```python
from build123d import *

# Parameters (mm, degrees)
IZIM1_W                     = 30
IZIM1_H                     = 20
Y_KSEKLIK_EKSTR_ZYON1_DEPTH = 3
Y_KSEKLIK_EKSTR_ZYON2_START = -10
Y_KSEKLIK_EKSTR_ZYON2_DEPTH = 3
Y_KSEKLIK_EKSTR_ZYON3_START = -16
Y_KSEKLIK_EKSTR_ZYON3_DEPTH = 3
IZIM3_R                     = 1
KES_EKSTR_ZYON1_DEPTH       = 25


with BuildPart() as part:
    # izim1 → Y_kseklik-Ekstr_zyon1 (new body)
    with BuildSketch(Plane.XY):
        with Locations((15, 10)):
            Rectangle(IZIM1_W, IZIM1_H)
    extrude(amount=Y_KSEKLIK_EKSTR_ZYON1_DEPTH)

    # izim2 → Y_kseklik-Ekstr_zyon2 (add)
    with BuildSketch(Plane.ZY.offset(Y_KSEKLIK_EKSTR_ZYON2_START)):
        with BuildLine():
            Line((3, 0), (3, 20))
            Line((3, 20), (19, 20))
            ThreePointArc((19, 20), (14.507810594, 7.193751525), (3, 0))
        make_face()
    extrude(amount=-Y_KSEKLIK_EKSTR_ZYON2_DEPTH)

    # izim2_2 → Y_kseklik-Ekstr_zyon3 (add)
    with BuildSketch(Plane.ZY.offset(Y_KSEKLIK_EKSTR_ZYON3_START)):
        with BuildLine():
            Line((3, 0), (3, 20))
            Line((3, 20), (19, 20))
            ThreePointArc((19, 20), (14.507810594, 7.193751525), (3, 0))
        make_face()
    extrude(amount=-Y_KSEKLIK_EKSTR_ZYON3_DEPTH)

    # izim3 → Kes-Ekstr_zyon1 (cut)
    with BuildSketch(Plane.ZY.offset(-10)):
        with Locations(Location((9.205520774, 11.392083612, 0), (0, 0, 180))):
            Circle(IZIM3_R)
    extrude(amount=-KES_EKSTR_ZYON1_DEPTH, mode=Mode.SUBTRACT)


solid = part.part
```
The model under review builds one solid part; all positions refer to its coordinate system, in mm. A direction names the side the tool comes from. Give positions to 0.01 mm unless a question says otherwise; leave off trailing zeros. Write each loop counter-clockwise with the first axis right and the second up, starting at its lowest first coordinate (ties: lowest second). Pieces come first, ordered by that corner, then holes.
(1) Consider section B-B, the plane y = 12. Give the boundary of the cut face in (x, z), and give its area (3 significant figures).
(2) For P1, Ø11, axis at x = 3.5, y = 8, coming from the +Z side; P2, Ø1, axis at y = 3.5, z = 4, coming from the -X side; P3, Ø1.2, axis at y = 11.39, z = 9.21, coming from the +X side; P4, Ø5, axis at y = 11, z = 13, coming from the +X side, all flat-tipped, find the tip position at first contact; note any pin that passes through.
(3) Consider section C-C, the plane x = 27. Give the boundary of the cut face in (y, z).
(4) To check wall thickness, follow L1, parallel to X at y = 5.5, z = 4.25; L2, parallel to Y at x = 12.75, z = 8.75; L3, parallel to Z at x = 11, y = 11.25. State the ranges of each line that lie inside material, in increasing order.
(5) Consider section A-A, the plane z = 17. Give the boundary of the cut face in (x, y).
(6) Tool access review of faces 1 (the flat face through (24, 10, 3)), 2 (the flat face through (10, 12, 11)), 3 (the cylindrical face through (17.479, 11.092, 8.252)), 4 (the flat face through (14, 10, 3)): name each direction out of +Z, -Z, +X, -X, +Y, -Y from which nothing blocks a thin tool from reaching the whole face with its end or side.
(7) Consider section D-D, the plane z = 4.75. Give the boundary of the cut face in (x, y), and give its area (3 significant figures).
(8) The part is to be moulded in two halves that separate along X. For faces 5 (the flat face through (5, 10, 3)), 6 (the flat face through (16, 12, 11)), 7 (the flat face through (0, 10, 1)), say which applies: released by +X, released by -X, zero draft, split by the parting line, or undercut.
Returned:
1. outline: (0, 0) - (30, 0) - (30, 3) - (19, 3) - (19, 8.41) - (16, 8.41) - (16, 3) - (13, 3) - (13, 8.41) - (10, 8.41) - (10, 3) - (0, 3) - close; (10, 10) - (13, 10) - (13, 17.37) - (10, 17.37) - close; (16, 10) - (19, 10) - (19, 17.37) - (16, 17.37) - close
1. area: 167 mm2
2. P1: stops at z = 3
2. P2: stops at x = 10
2. P3: passes through
2. P4: stops at x = 19
3. outline: (0, 0) - (20, 0) - (20, 3) - (0, 3) - close
4. L1: x = 10 to 13, 16 to 19
4. L2: y = 2.25 to 10.5, 12.28 to 20
4. L3: z = 0 to 8.22, 10.2 to 17.04
5. outline: (10, 11.17) - (13, 11.17) - (13, 20) - (10, 20) - close; (16, 11.17) - (19, 11.17) - (19, 20) - (16, 20) - close
6. face 1: +Z, +X, +Y, -Y
6. face 2: +Z, -X, +Y, -Y
6. face 3: +X, -X
6. face 4: +Z, +Y, -Y
7. outline: (10, 0.48) - (13, 0.48) - (13, 20) - (10, 20) - close; (16, 0.48) - (19, 0.48) - (19, 20) - (16, 20) - close
7. area: 117 mm2
8. face 5: zero draft
8. face 6: undercut
8. face 7: released by -X
